Could you check a few things on this model? Use its own coordinates, in mm. A direction names the side the tool comes from. Give positions to 0.01 mm unless a question says otherwise; leave off trailing zeros. Loops run counter-clockwise (first coordinate to the right, second up) from the corner with the lowest first, then second, coordinate; pieces in that order, holes last. Notation, with made-up numbers: M 85.25,9 L 110.25,9 A24 ccw 110.25,22 Z; hole C 33.5,76 d1. An arc over 180 degrees is marked long. Use CSV: the item, a comma, the result in double quotes.
```python
from build123d import *

# Parameters (mm, degrees)
EXTRUDE_1_DEPTH     = 20
SKETCH_2_W          = 15
SKETCH_2_H          = 10
EXTRUDE_2_DEPTH     = 10
SKETCH_3_W          = 50
SKETCH_3_H          = 10
EXTRUDE_3_DEPTH     = 5
EXTRUDE_4_DEPTH     = 10
CUT_EXTRUDE_2_DEPTH = 82.631660278
EXTRUDE_5_DEPTH     = 10


with BuildPart() as part:
    # 草图1 → 凸台-拉伸1 (new body)
    with BuildSketch(Plane(origin=(0, 0, 0), x_dir=(1, 0, 0), z_dir=(0, 1, 0))):
        Polygon((0, 0), (0, -15), (70, -30), (70, 0), align=None)
    extrude(amount=EXTRUDE_1_DEPTH)

    # 草图2 → 凸台-拉伸2 (add)
    with BuildSketch(Plane(origin=(0, 20, 0), x_dir=(1, 0, 0), z_dir=(0, 1, 0))):
        with Locations((62.5, -15)):
            Rectangle(SKETCH_2_W, SKETCH_2_H)
    extrude(amount=EXTRUDE_2_DEPTH)

    # 草图3 → 凸台-拉伸3 (add)
    with BuildSketch(Plane(origin=(0, 20, 0), x_dir=(1, 0, 0), z_dir=(0, 1, 0))):
        with Locations((45, -5)):
            Rectangle(SKETCH_3_W, SKETCH_3_H)
    extrude(amount=EXTRUDE_3_DEPTH)

    # 草图6 → 凸台-拉伸4 (add)
    with BuildSketch(Plane(origin=(0, 0, 20), x_dir=(-1, 0, 0), z_dir=(0, 0, -1))):
        Polygon((-23.333333333, 20), (-55, 30), (-55, 20), align=None)
    extrude(amount=EXTRUDE_4_DEPTH)

    # 草图12 → 切除-拉伸2 (cut, through all)
    with BuildSketch(Plane(origin=(-3.62720403, 11.486146096, 0), x_dir=(0.9535826651341409, 0.30113136793709994, 0), z_dir=(-0.3011313679370999, 0.9535826651341408, 0))):
        Polygon((2.464685971, 0), (2.464685971, -20), (63.372000863, -20), (63.372000863, -10), (25.094280661, -10), (25.094280661, 0), align=None)
    extrude(amount=CUT_EXTRUDE_2_DEPTH, mode=Mode.SUBTRACT)

    # 草图14 → 凸台-拉伸5 (add)
    with BuildSketch(Plane.XY.offset(10)):
        Polygon((20, 20), (20, 18.947368421), (20.304276784, 19.043455826), align=None)
    extrude(amount=-EXTRUDE_5_DEPTH)


solid = part.part
```
1. I want a section at C-C, the plane z = 10.75. List the corners of the cut face in (x, y) for me, then the cut area to 3 significant figures.
Outcome:
outline,"M 0,0 L 70,0 L 70,30 L 55,30 L 0,12.63 Z"
area,"1,620 mm2"
2. I want a section at A-A, the plane x = 40. List the corners of the cut face in (y, z) for me.
Outcome:
outline,"M 0,0 L 25,0 L 25,10 L 25.26,10 L 25.26,20 L 20,20 L 20,23.57 L 0,23.57 Z"
3. Please list where these lines run through material, in increasing order: line 1 (Z direction, x = 30.5, y = 23.25); line 2 (Y direction, x = 45, z = 23).
Outcome:
line 1,"0 to 10"
line 2,"0 to 20"
4. I'm going to push flat-ended pins straight in: pin 1 Ø1.5 at (x, y) = (60, 21.5) entering from +Z; pin 2 Ø5 at (x, z) = (16, 5) entering from +Y; pin 3 Ø6.5 at (x, y) = (25, 22.5) entering from +Z. Where does each tip first touch, or does it pass through?
Outcome:
pin 1,"z = 20"
pin 2,"y = 18.47"
pin 3,"z = 20.8"
5. Which directions (+Z, -Z, +X, -X, +Y, -Y) give clear straight access to the entire face, cutting with the end or side of a thin tool? Please do faces 1 (the face through (35, 13, 0)), 2 (the face through (57, 20, 23)), 3 (the face through (27, 23, 10)), 4 (the face through (58, 28, 10)), 5 (the face through (20, 22, 5)).
Outcome:
face 1,"-Z, +X, -X, +Y, -Y"
face 2,"+Z, +X, -X, +Y"
face 3,"+Z, -X, +Y"
face 4,"-Z, +X, -X, +Y"
face 5,"+Z, -Z, -X, +Y"
6. I want a section at B-B, the plane y = 7. List the corners of the cut face in (x, z) for me, then the cut area to 4 significant figures.
Outcome:
outline,"M 0,0 L 70,0 L 70,30 L 0,15 Z"
area,"1,575 mm2"
7. I want a section at D-D, the plane y = 22.5. List the corners of the cut face in (x, z) for me.
Outcome:
outline,"M 20,0 L 70,0 L 70,20 L 31.25,20 L 31.25,10 L 20,10 Z"
